Autodesk Inventor part; units mm, degrees
ref_plane "Work Plane2" through (-36.5132, 1.6, 47.4786) normal (0, 1, 0) x (1, 0, 0)
ref_plane "YZ Plane" through (0, 0, 0) normal (1, 0, 0) x (0, 1, 0)
ref_plane "XZ Plane" through (0, 0, 0) normal (0, 1, 0) x (-1, 0, 0)
ref_plane "Work Plane2" through (-36.5132, 1.6, 47.4786) normal (0, 1, 0) x (1, 0, 0)
sketch "Sketch1" plane through (-36.5132, 1.6, 47.4786) normal (0, 1, 0) x (1, 0, 0)
  line L0 (-22.6989, -29.8949) -> (32.3011, -29.8949)
  line L1 (37.3011, -24.8949) -> (37.3011, 69.1051)
  line L2 (32.3011, 74.1051) -> (-22.6989, 74.1051)
  line L3 (-27.6989, 69.1051) -> (-27.6989, -24.8949)
  arc A0 (-27.6989, -24.8949) -> (-22.6989, -29.8949) centre (-22.6989, -24.8949) ccw
  arc A1 (-22.6989, 74.1051) -> (-27.6989, 69.1051) centre (-22.6989, 69.1051) ccw
  arc A2 (37.3011, 69.1051) -> (32.3011, 74.1051) centre (32.3011, 69.1051) ccw
  arc A3 (32.3011, -29.8949) -> (37.3011, -24.8949) centre (32.3011, -24.8949) ccw
  line L4 (-22.6989, -24.8949) -> (32.3011, -24.8949) construction
  line L5 (32.3011, -24.8949) -> (32.3011, 69.1051) construction
  line L6 (32.3011, 69.1051) -> (-22.6989, 69.1051) construction
  line L7 (-22.6989, 69.1051) -> (-22.6989, -24.8949) construction
  dimension "d2" = 5
  dimension "d5" = 94
  dimension "d6" = 55
extrude "Extrusion1" add sketch "Sketch1" along normal blind 3
sketch "Sketch2" plane through (-36.5132, 1.6, 47.4786) normal (0, -1, 0) x (1, 0, 0)
  arc A0 (-22.6989, 29.8949) -> (-27.6989, 24.8949) centre (-22.6989, 24.8949) ccw construction
  arc A1 (-27.6989, -69.1051) -> (-22.6989, -74.1051) centre (-22.6989, -69.1051) ccw construction
  arc A2 (32.3011, -74.1051) -> (37.3011, -69.1051) centre (32.3011, -69.1051) ccw construction
  arc A3 (37.3011, 24.8949) -> (32.3011, 29.8949) centre (32.3011, 24.8949) ccw construction
hole "Hole1" at (-59.2121, 1.6, -21.6265) at (-4.2121, 1.6, 72.3735) at (-59.2121, 1.6, 72.3735) at (-4.2121, 1.6, -21.6265) direction (0, 1, 0) diameter 3.2766 end through all
equation "\"d5\" = LCD_PCB_Horizontal_Hole_Spacing"
equation "\"d6\" = LCD_PCB_Vertical_Hole_Spacing"
properties part number "LCD_Cover" material "Polycarbonate, Clear"
Source: CAD feature listing. Evaluate the final solid. Frame: model axes, mm. Give positions to 0.01 mm unless a question says otherwise; leave off trailing zeros. Answer as a JSON object with one key per item and string values.
Q1. Ray query, line 1 along X through (y, z) = (2.2, 71); line 2 along Z through (x, y) = (-58, 4.4); line 3 along Z through (x, y) = (-61, 3). Return the intervals inside material, ascending.
Geometry check:
{"line 1": "x = -64.21 to -60.11, -58.32 to -5.11, -3.32 to 0.79", "line 2": "z = -26.63 to -22.73, -20.52 to 71.27, 73.48 to 77.37", "line 3": "z = -26.3 to 77.04"}
Q2. Contact query for flat-ended pins moving along their axis: P1, Ø2.5, axis at x = -59.21, z = -21.63, coming from the -Y side; P2, Ø4, axis at x = -4.21, z = -21.63, coming from the -Y side. Output: stop coordinate, or through.
Geometry check:
{"P1": "passes through", "P2": "stops at y = 1.6"}
Q3. Mould query, pull axis X, two halves, no side actions, for faces 1 (the face through (0.788, 3, 26)), 2 (the face through (-31, 3, -26.626)), 3 (the face through (-60.6, 3.1, 71.5)). Classes: +X half, -X half, draft (parallel to the pull), parting line (faces both ways), or undercut.
Geometry check:
{"face 1": "+X half", "face 2": "draft", "face 3": "undercut"}
